from build123d import *

# Parameters (mm, degrees)
SKETCH1_R           = 73.66
BOSS_EXTRUDE1_DEPTH = 6.35
CUT_EXTRUDE1_DEPTH  = 7.35
SKETCH4_R           = 4.7625
CUT_EXTRUDE2_DEPTH  = 7.35


with BuildPart() as part:
    # Sketch1 → Boss-Extrude1 (new body)
    with BuildSketch(Plane.XY):
        Circle(SKETCH1_R)
    extrude(amount=BOSS_EXTRUDE1_DEPTH)

    # Sketch2 → Cut-Extrude1 (cut, through all)
    with BuildSketch(Plane(origin=(0, 0, 0), x_dir=(-1, 0, 0), z_dir=(0, 0, -1))):
        Polygon((-48.26, 0), (-48.26, 3.175), (-76.2, 3.175), (-76.2, -3.175), (-48.26, -3.175), align=None)
        Polygon((48.26, -3.175), (48.26, 0), (48.26, 3.175), (76.2, 3.175), (76.2, -3.175), align=None)
    extrude(amount=-CUT_EXTRUDE1_DEPTH, mode=Mode.SUBTRACT)

    # Sketch4 → Cut-Extrude2 (cut, through all)
    with BuildSketch(Plane(origin=(0, 0, 0), x_dir=(-1, 0, 0), z_dir=(0, 0, -1))):
        with Locations((0, -59.3725)):
            Circle(SKETCH4_R)
        with Locations((0, 59.3725)):
            Circle(SKETCH4_R)
    extrude(amount=-CUT_EXTRUDE2_DEPTH, mode=Mode.SUBTRACT)


solid = part.part
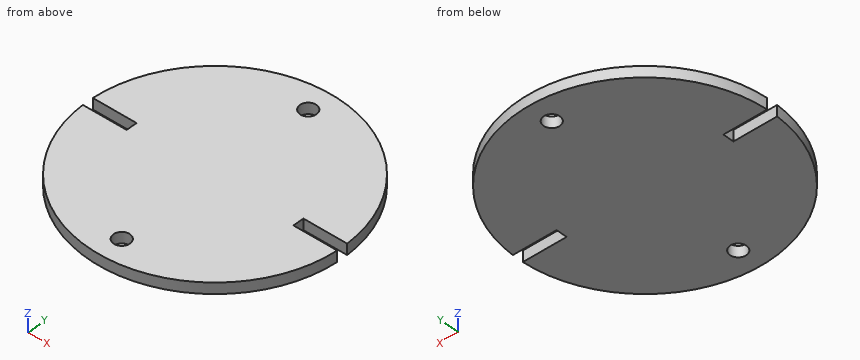
Source: CAD feature listing. Evaluate the final solid. Frame: model axes, mm. Give positions to 0.01 mm unless a question says otherwise; leave off trailing zeros. Loops run counter-clockwise (first coordinate to the right, second up) from the corner with the lowest first, then second, coordinate; pieces in that order, holes last. Notation, with made-up numbers: (-28, -9) -> (-6, -9) arc R33 cw to (-6, 21) -> close; hole circle Ø10 at (53, 77). An arc over 180 degrees is marked (long way). Use a Markdown table: item, result. Add a question column.
1) Section query C-C, the plane y = 0. Return the cut outline in (x, z), then the cut area to 3 significant figures.
2) Section query A-A, the plane x = 0. Return the cut outline in (y, z) (3 decimals), then the cut area to 3 significant figures.
3) Section query D-D, the plane x = -21. Return the cut outline in (y, z), then the cut area to 3 significant figures.
4) Line query: line 1 along Y through (x, z) = (0, 3.5) (3 decimals); line 2 along Y through (x, z) = (-2, 4); line 3 along Y through (x, z) = (-65, 3.5) (1 decimal). Output: solid intervals per line, ascending. Write a range as [from, to].
5) First-contact query: pin 1 (1 mm diameter, centred on x = 23.5, z = 3, fed in from -Y); pin 2 (2 mm diameter, centred on y = 27, z = 3.5, fed in from +X); pin 3 (1 mm diameter, centred on y = 52.5, z = 4.5, fed in from +X). Flat tips, straight axial feed; report the tip coordinate or a pass-through.
Numbers:
| question | item | result |
|---|---|---|
| 1 | outline | (-48.26, 0) -> (48.26, 0) -> (48.26, 6.35) -> (-48.26, 6.35) -> close |
| 1 | area | 613 mm2 |
| 2 | outline | (-73.66, 0) -> (-64.135, 0) -> (-64.135, 6.35) -> (-73.66, 6.35) -> close; (-54.61, 0) -> (54.61, 0) -> (54.61, 6.35) -> (-54.61, 6.35) -> close; (64.135, 0) -> (73.66, 0) -> (73.66, 6.35) -> (64.135, 6.35) -> close |
| 2 | area | 815 mm2 |
| 3 | outline | (-70.6, 0) -> (70.6, 0) -> (70.6, 6.35) -> (-70.6, 6.35) -> close |
| 3 | area | 897 mm2 |
| 4 | line 1 | y = [-73.66, -64.135], [-54.61, 54.61], [64.135, 73.66] |
| 4 | line 2 | y = [-73.63, -63.69], [-55.05, 55.05], [63.69, 73.63] |
| 4 | line 3 | y = [-34.7, -3.2], [3.2, 34.7] |
| 5 | pin 1 | stops at y = -69.98 |
| 5 | pin 2 | stops at x = 68.92 |
| 5 | pin 3 | stops at x = 52.17 |
